Part print with two shaded views. Sizes in mm from the minimum x, y, z corner. A direction names the side the tool comes from. Give positions to 0.01 mm unless a question says otherwise; leave off trailing zeros. Loops run counter-clockwise (first coordinate to the right, second up) from the corner with the lowest first, then second, coordinate; pieces in that order, holes last. Notation, with made-up numbers: (4.25, 77) -> (33.25, 77) arc R27 ccw to (33.25, 112) -> close; hole circle Ø6 at (-35, 77.25). An arc over 180 degrees is marked (long way). One line per question, with ' | ' between items. Start each with the question number.
(1) Slice it at C-C, the plane z = 28. Write the cut outline in (x, y) (1 decimal).
(2) 3-axis set-ups, long thin cutter, end or side, ignore diameter. For the marked faces 1, 2, 3, 4 and 5: which of +Z, -Z, +X, -X, +Y, -Y reach the whole face in a straight line?
(3) Slice it at D-D, the plane x = 8.5. Write the cut outline in (y, z) (1 decimal).
(4) Slice it at B-B, the plane y = 1.85. Write the cut outline in (x, z).
(5) Drill centre lines: L1, parallel to Z at x = 6.5, y = 1.4; L2, parallel to X at y = 3.7, z = 28.85; L3, parallel to X at y = 2.4, z = 3.2. Where is each one in solid material? Low to high. Write a range as from..to.
(6) Mould opens along X. For the marked faces 6, 7 and 8 say: pulls with the +X half, pulls with the -X half, needs draft (parallel to the pull), parting line crosses it, or undercut.
(7) Flat gauge pins, fed straight in: pin 1 Ø4 at (x, z) = (6.5, 31) entering from +Y; pin 2 Ø7 at (x, z) = (5.5, 2) entering from +Y; pin 3 Ø0.5 at (x, y) = (8, 5) entering from -Z. Where does each tip first touch, or does it go through?
(8) Slice it at A-A, the plane x = 6.5. Write the cut outline in (y, z).
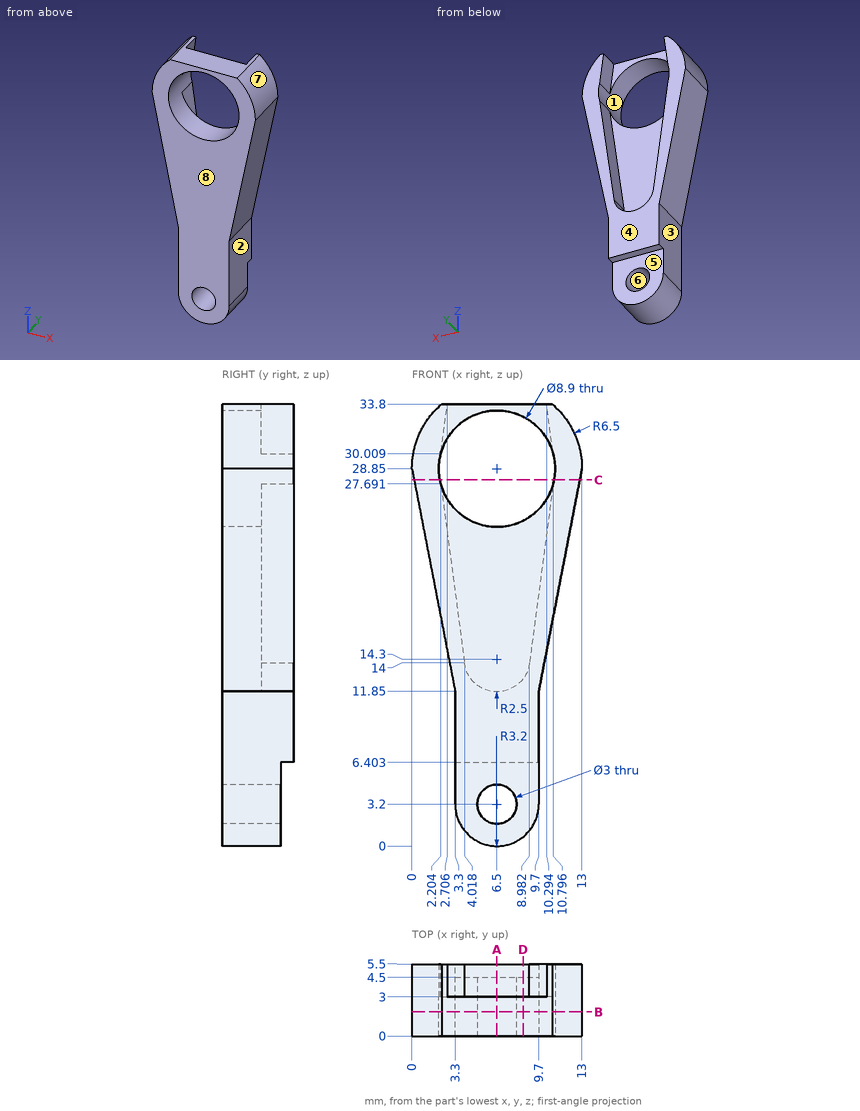
Final values:
1) outline: (0.2, 0) -> (2.1, 0) -> (2.1, 5.5) -> (0.2, 5.5) -> close; (10.9, 0) -> (12.8, 0) -> (12.8, 5.5) -> (10.9, 5.5) -> close
2) face 1: +Y, -Y | face 2: -Z, +X, +Y, -Y | face 3: -Z, -X, +Y, -Y | face 4: +Z, -Z, +X, -X, +Y | face 5: -Z, +X, -X, +Y
3) outline: (0, 0.7) -> (4.5, 0.7) -> (4.5, 6.4) -> (5.5, 6.4) -> (5.5, 12.8) -> (3, 12.8) -> (3, 24.9) -> (0, 24.9) -> close; (0, 32.8) -> (3, 32.8) -> (3, 33.8) -> (0, 33.8) -> close
4) outline: (0, 28.85) -> (3.3, 11.85) -> (3.3, 3.2) arc R3.2 ccw to (9.7, 3.2) -> (9.7, 11.85) -> (13, 28.85) arc R6.5 ccw to (10.71, 33.8) -> (2.29, 33.8) arc R6.5 ccw to start; hole circle Ø8.9 at (6.5, 28.85); hole circle Ø3 at (6.5, 3.2)
5) L1: 0..1.7, 4.7..24.4, 33.3..33.8 | L2: 0..2.05, 10.95..13 | L3: 3.3..5, 8..9.7
6) face 6: undercut | face 7: pulls with the +X half | face 8: needs draft
7) pin 1: through | pin 2: y = 4.5 | pin 3: z = 6.4
8) outline: (0, 0) -> (4.5, 0) -> (4.5, 1.7) -> (0, 1.7) -> close; (0, 4.7) -> (4.5, 4.7) -> (4.5, 6.4) -> (5.5, 6.4) -> (5.5, 11.8) -> (3, 11.8) -> (3, 24.4) -> (0, 24.4) -> close; (0, 33.3) -> (3, 33.3) -> (3, 33.8) -> (0, 33.8) -> close
